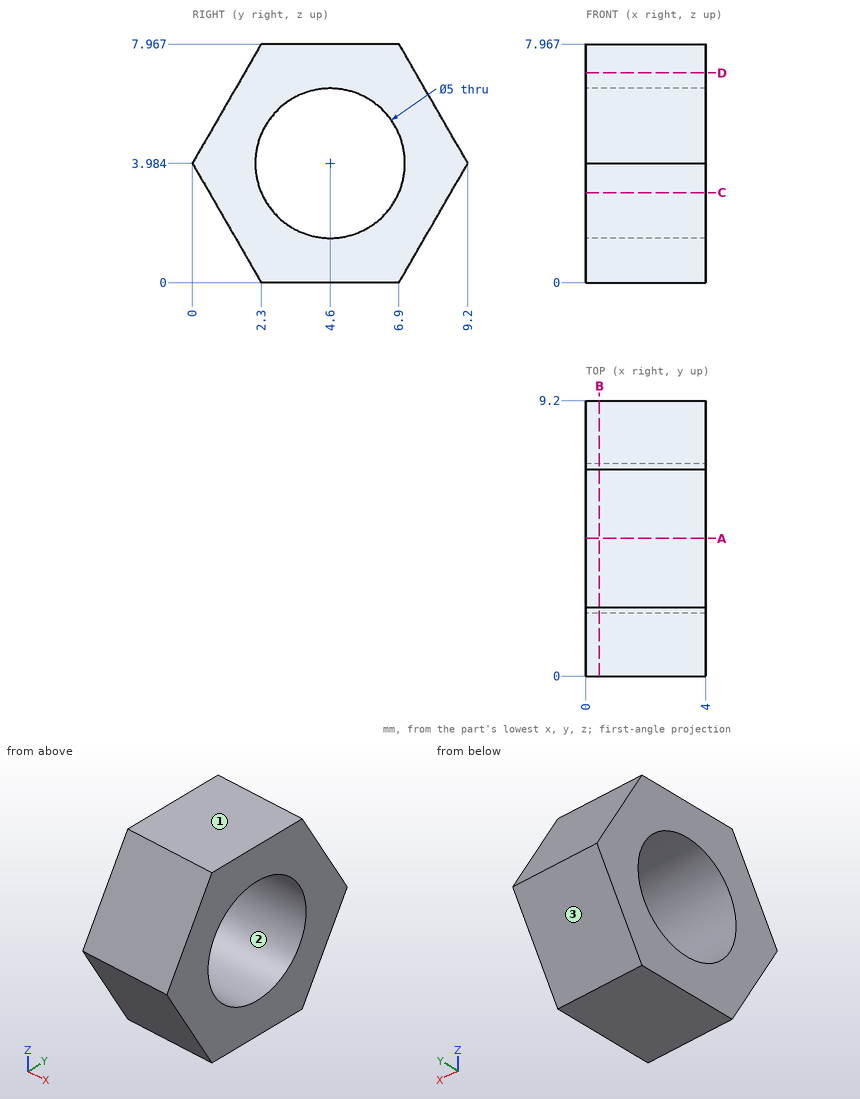
Can you work these out from the drawing? Everything is in mm from the part's minimum corner. Coordinates: 2 decimals unless noted, no trailing zeros. Loops run counter-clockwise (first coordinate to the right, second up) from the corner with the lowest first, then second, coordinate; pieces in that order, holes last. Notation, with made-up numbers: M 69,9 L 111,9 A22 ccw 111,35 Z; hole C -29.75,-24 d11. An arc over 180 degrees is marked long. One line per item, written item: value.
1. Please list where these lines run through material, in increasing order: probe 1 along Z at (x, y) = (2.2, 4.6); probe 2 along Y at (x, z) = (0.5, 3.25) (1 decimal); probe 3 along Y at (x, z) = (0.35, 3.75) (1 decimal).
Geometry says:
probe 1: z = 0 to 1.48, 6.48 to 7.97
probe 2: y = 0.4 to 2.2, 7 to 8.8
probe 3: y = 0.1 to 2.1, 7.1 to 9.1
2. Imagine slicing it at B-B (x = 0.45). List the corners of the cut face in (y, z) for me.
Geometry says:
outline: M 0,3.98 L 2.3,0 L 6.9,0 L 9.2,3.98 L 6.9,7.97 L 2.3,7.97 Z; hole C 4.6,3.98 d5
3. Imagine slicing it at D-D (z = 7). List the corners of the cut face in (x, y) for me, and give its area (3 significant figures).
Geometry says:
outline: M 0,1.74 L 4,1.74 L 4,7.46 L 0,7.46 Z
area: 22.9 mm2
4. Will this pin go through, and if not, where does the flat tip stop? pin 1 Ø1.5 at (x, z) = (2.5, 2) entering from -Y.
Geometry says:
pin 1: stops at y = 0.71
5. Imagine slicing it at A-A (y = 4.6). List the corners of the cut face in (x, z) for me.
Geometry says:
outline: M 0,0 L 4,0 L 4,1.48 L 0,1.48 Z; M 0,6.48 L 4,6.48 L 4,7.97 L 0,7.97 Z
6. Imagine slicing it at C-C (z = 3). List the corners of the cut face in (x, y) for me, and give its area (3 significant figures).
Geometry says:
outline: M 0,0.57 L 4,0.57 L 4,2.3 L 0,2.3 Z; M 0,6.9 L 4,6.9 L 4,8.63 L 0,8.63 Z
area: 13.9 mm2
7. Thinking about a two-plate mould opening in Y: for the marked faces 1, 2 and 3, which applies, +Y half, -Y half, draft (parallel to the pull), parting line (faces both ways), or undercut?
Geometry says:
face 1: draft
face 2: undercut
face 3: +Y half
